```python
from build123d import *

# Parameters (mm, degrees)
SKETCH1_R           = 7.75
SKETCH1_R_2         = 3
BOSS_EXTRUDE3_DEPTH = 3
BOSS_EXTRUDE4_START = -6
SKETCH3_R           = 3
SKETCH3_R_2         = 1.7025
BOSS_EXTRUDE4_DEPTH = 6
CUT_EXTRUDE1_DEPTH  = 0.5


with BuildPart() as part:
    # Sketch1 → Boss-Extrude3 (new body)
    with BuildSketch(Plane.XY):
        with BuildLine():
            Line((8.434915556, -5.371424351), (21.165047264, 14.249110995))
            ThreePointArc((21.165047264, 14.249110995), (21.364152327, 19.357269814), (16.970562748, 21.970562748))
            Line((16.970562748, 21.970562748), (-17.47367286, 22.673506332))
            ThreePointArc((-17.47367286, 22.673506332), (-22.032126076, 20.135047844), (-21.848877926, 14.920674696))
            Line((-21.848877926, 14.920674696), (-8.342416793, -5.513989668))
            ThreePointArc((-8.342416793, -5.513989668), (0.084971894, -9.999638982), (8.434915556, -5.371424351))
        make_face()
        Circle(SKETCH1_R, mode=Mode.SUBTRACT)
        with Locations((-17.67766953, 17.67766953)):
            Circle(SKETCH1_R_2, mode=Mode.SUBTRACT)
        with Locations((16.970562748, 16.970562748)):
            Circle(SKETCH1_R_2, mode=Mode.SUBTRACT)
    extrude(amount=BOSS_EXTRUDE3_DEPTH)

    # Sketch3 → Boss-Extrude4 (add)
    # profile 1 of 2: a face of its own
    with BuildSketch(Plane.XY.offset(3).offset(BOSS_EXTRUDE4_START)):
        with Locations((-17.67766953, 17.67766953)):
            Circle(SKETCH3_R)
        with Locations((-17.67766953, 17.67766953)):
            Circle(SKETCH3_R_2, mode=Mode.SUBTRACT)
    # profile 2 of 2: a face of its own
    with BuildSketch(Plane.XY.offset(3).offset(BOSS_EXTRUDE4_START)):
        with Locations((16.970562748, 16.970562748)):
            Circle(SKETCH3_R)
        with Locations((16.970562748, 16.970562748)):
            Circle(SKETCH3_R_2, mode=Mode.SUBTRACT)
    extrude(amount=BOSS_EXTRUDE4_DEPTH)

    # Sketch4 → Cut-Extrude1 (cut)
    with BuildSketch(Plane.XY.offset(3)):
        Polygon((-0.501047916, 14.710849075), (0.127157212, 14.710849075), (0.127157212, 11.839054203), (1.1143367, 11.839054203), (1.1143367, 11.210849075), (-0.501047916, 11.210849075), align=None)
    extrude(amount=-CUT_EXTRUDE1_DEPTH, mode=Mode.SUBTRACT)


solid = part.part
```
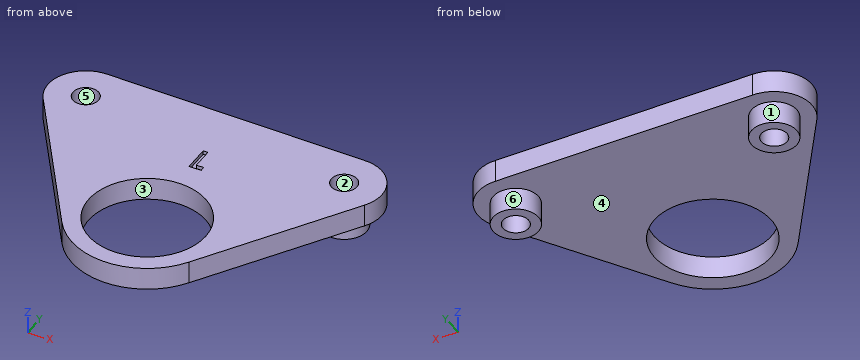
Design review of the part built by this model. Coordinates are the model's own, in mm. Face numbers are marked on the shaded views. A direction names the side the tool comes from. Coordinates: 2 decimals unless noted, no trailing zeros. Loops run counter-clockwise (first coordinate to the right, second up) from the corner with the lowest first, then second, coordinate; pieces in that order, holes last. Notation, with made-up numbers: (84, 87.5) - (107, 87.5) arc R27 ccw to (107, 115.5) - close; hole circle Ø5 at (40.5, 72.5). An arc over 180 degrees is marked (long way). Use CSV: the item, a comma, the result in double quotes. Start each with the question number.
1) Consider section B-B on x = 5. Write out the cut boundary in (y, z).
2) Tool access review of the marked faces 5 and 6: name each direction out of +Z, -Z, +X, -X, +Y, -Y from which nothing blocks a thin tool from reaching the whole face with its end or side.
3) Consider section C-C on z = 2.05. Give the number of separate pieces and of enclosed holes in the cut face, then the cut area to 3 significant figures.
4) Wall thickness on L1, parallel to X at y = 17, z = -1.6; L2, parallel to X at y = 18, z = -0.65; L3, parallel to Z at x = -10.5, y = 15.5: over which ranges is each line inside the solid? List them lowest first. Write a range as from..to.
5) Consider section D-D on x = -15.5. Write out the cut boundary in (y, z), then the cut area to 3 significant figures.
6) The part is to be moulded in two halves that separate along Y. For the marked faces 1, 2, 3 and 4, say which applies: +Y half, -Y half, draft (parallel to the pull), parting line (faces both ways), or undercut.
7) Consider section A-A on y = 0. Write out the cut boundary in (x, z).
8) For pin 1 Ø0.6 at (y, z) = (11.5, 2.5) entering from -X; pin 2 Ø4 at (x, y) = (16.97, 16.97) entering from -Z; pin 3 Ø1 at (x, z) = (13.5, 0) entering from -Y; pin 4 Ø3 at (y, z) = (7.5, -1) entering from -X, all flat-tipped, find the tip position at first contact; note any pin that passes through.
Geometry says:
1,outline,"(-8.66, 0) - (-5.92, 0) - (-5.92, 3) - (-8.66, 3) - close; (5.92, 0) - (22.21, 0) - (22.21, 3) - (5.92, 3) - close"
2,face 5,"+Z, -Z"
2,face 6,"-Z"
3,separate pieces,"1"
3,enclosed holes,"3"
3,area,"779 mm^2"
4,L1,"-20.6..-19.24, -16.12..-14.76, 13.97..15.27, 18.67..19.97"
4,L2,"-20.66..-19.35, -16.01..-14.7, 14.15..15.61, 18.33..19.79"
4,L3,"0..3"
5,outline,"(5.32, 0) - (15.61, 0) - (15.61, -3) - (19.74, -3) - (19.74, 0) - (22.63, 0) - (22.63, 3) - (5.32, 3) - close"
5,area,"64.3 mm^2"
6,face 1,"parting line"
6,face 2,"undercut"
6,face 3,"undercut"
6,face 4,"draft"
7,outline,"(-11.99, 0) - (-7.75, 0) - (-7.75, 3) - (-11.99, 3) - close; (7.75, 0) - (11.92, 0) - (11.92, 3) - (7.75, 3) - close"
8,pin 1,"x = -19.79"
8,pin 2,"z = -3"
8,pin 3,"y = 1.66"
8,pin 4,"x = -17.68"
